Geometry check sheet. Reference: the model listing, model coordinates, mm. A direction names the side the tool comes from. Give positions to 0.01 mm unless a question says otherwise; leave off trailing zeros. Order: outer loops, then holes, each group sorted by start corner. A loop starts at its lowest first (then second) coordinate and runs counter-clockwise, first axis right, second up. Notation, with made-up numbers: M 65,11 L 80,11 A23 cw 80,40 Z; hole C -18.75,-27.75 d11. An arc over 180 degrees is marked long. Answer as a JSON object with one key per item and string values. Group by question number.
from build123d import *

# Parameters (mm, degrees)
SKETCH1_W            = 72
SKETCH1_H            = 125
BOSS_EXTRUDE1_DEPTH  = 2
SKETCH5_W            = 72
SKETCH5_H            = 2
BOSS_EXTRUDE3_DEPTH  = 35
SKETCH6_W            = 2
SKETCH6_H            = 125
BOSS_EXTRUDE4_DEPTH  = 35
SKETCH7_W            = 5
SKETCH7_H            = 5
BOSS_EXTRUDE5_DEPTH  = 35
FILLET2_R            = 1.5
SKETCH8_R            = 2.375
CUT_EXTRUDE2_DEPTH   = 92.049437121
FILLET2_OF_MIRROR4_R = 1.5
FILLET3_R            = 2
SKETCH12_W           = 68
SKETCH12_H           = 2
BOSS_EXTRUDE6_DEPTH  = 35
SKETCH13_W           = 5
SKETCH13_H           = 5
BOSS_EXTRUDE9_DEPTH  = 35
SKETCH14_R           = 2.375
CUT_EXTRUDE6_DEPTH   = 92.049437121
FILLET4_R            = 1.5
FILLET4_OF_MIRROR8_R = 1.5


with BuildPart() as part:
    # Sketch1 → Boss-Extrude1 (new body)
    with BuildSketch(Plane.XY):
        with Locations((0, -12.5)):
            Rectangle(SKETCH1_W, SKETCH1_H)
    extrude(amount=BOSS_EXTRUDE1_DEPTH)

    # Sketch5 → Boss-Extrude3 (add)
    with BuildSketch(Plane.XY.offset(2)):
        with Locations((0, 49)):
            Rectangle(SKETCH5_W, SKETCH5_H)
    extrude(amount=BOSS_EXTRUDE3_DEPTH)

    # Sketch6 → Boss-Extrude4 (add)
    with BuildSketch(Plane.XY.offset(2)):
        with Locations((-35, -12.5)):
            Rectangle(SKETCH6_W, SKETCH6_H)
    boss_extrude4 = extrude(amount=BOSS_EXTRUDE4_DEPTH)

    # Mirror2: Boss-Extrude4 across plane
    add(boss_extrude4.mirror(Plane(origin=(0, 0, 0), x_dir=(0, 0, 1), z_dir=(1, 0, 0))))

    # Sketch7 → Boss-Extrude5 (add)
    with BuildSketch(Plane.XY.offset(2)):
        with Locations((-31.5, 45.5)):
            Rectangle(SKETCH7_W, SKETCH7_H)
    boss_extrude5 = extrude(amount=BOSS_EXTRUDE5_DEPTH)

    # Fillet2
    fillet2_edges = [part.edges().sort_by_distance(p)[0] for p in [
        (-29, 43, 19.5),
    ]]
    fillet(fillet2_edges, radius=FILLET2_R)

    # Sketch8 → Cut-Extrude2 (cut, through all)
    with BuildSketch(Plane.XY.offset(37)):
        with Locations((-32.2, 46.2)):
            Circle(SKETCH8_R)
    cut_extrude2 = extrude(amount=-CUT_EXTRUDE2_DEPTH, mode=Mode.SUBTRACT)

    # Mirror4: Boss-Extrude5, Cut-Extrude2 across plane
    add(boss_extrude5.mirror(Plane(origin=(0, 0, 0), x_dir=(0, 0, 1), z_dir=(1, 0, 0))))
    add(cut_extrude2.mirror(Plane(origin=(0, 0, 0), x_dir=(0, 0, 1), z_dir=(1, 0, 0))), mode=Mode.SUBTRACT)

    # Fillet2 of Mirror4
    fillet2_of_mirror4_edges = [part.edges().sort_by_distance(p)[0] for p in [
        (29, 43, 19.5),
    ]]
    fillet(fillet2_of_mirror4_edges, radius=FILLET2_OF_MIRROR4_R)

    # Fillet3
    fillet3_edges = [part.edges().sort_by_distance(p)[0] for p in [
        (-36, 50, 18.5),
        (36, 50, 18.5),
        (-36, -75, 18.5),
        (36, -75, 18.5),
    ]]
    fillet(fillet3_edges, radius=FILLET3_R - 0.0001)  # a hair under: the kernel refuses the full size

    # Sketch12 → Boss-Extrude6 (add)
    with BuildSketch(Plane.XY.offset(2)):
        with Locations((0, -74)):
            Rectangle(SKETCH12_W, SKETCH12_H)
    extrude(amount=BOSS_EXTRUDE6_DEPTH)

    # Sketch13 → Boss-Extrude9 (add)
    with BuildSketch(Plane.XY.offset(37)):
        with Locations((-31.5, -70.5)):
            Rectangle(SKETCH13_W, SKETCH13_H)
    boss_extrude9 = extrude(amount=-BOSS_EXTRUDE9_DEPTH)

    # Sketch14 → Cut-Extrude6 (cut, through all)
    with BuildSketch(Plane.XY.offset(37)):
        with Locations((-32.2, -71.2)):
            Circle(SKETCH14_R)
    cut_extrude6 = extrude(amount=-CUT_EXTRUDE6_DEPTH, mode=Mode.SUBTRACT)

    # Fillet4
    fillet4_edges = [part.edges().sort_by_distance(p)[0] for p in [
        (-29, -68, 19.5),
    ]]
    fillet(fillet4_edges, radius=FILLET4_R)

    # Mirror8: Boss-Extrude9, Cut-Extrude6 across plane
    add(boss_extrude9.mirror(Plane(origin=(0, 0, 0), x_dir=(0, 0, 1), z_dir=(1, 0, 0))))
    add(cut_extrude6.mirror(Plane(origin=(0, 0, 0), x_dir=(0, 0, 1), z_dir=(1, 0, 0))), mode=Mode.SUBTRACT)

    # Fillet4 of Mirror8
    fillet4_of_mirror8_edges = [part.edges().sort_by_distance(p)[0] for p in [
        (29, -68, 19.5),
    ]]
    fillet(fillet4_of_mirror8_edges, radius=FILLET4_OF_MIRROR8_R)


solid = part.part
1. Cross-section at C-C (z = 23). Record the cut outline in (x, y) (3 decimals), and give its area (3 significant figures).
2. Release check for a two-part mould opening along X. For faces 1 (the flat face through (-36, -13, 18)), 2 (the flat face through (36, -13, 18)), 3 (the cylindrical face through (30.92, -69.2, 18.76)), 4 (the flat face through (0, 50, 18)) record: released by +X, released by -X, zero draft, split by the parting line, or undercut.
3. Cross-section at B-B (x = 32.2). Record the cut outline in (y, z) (3 decimals).
4. Cross-section at D-D (x = 20). Record the cut outline in (y, z).
5. Access from +Z, -Z, +X, -X, +Y, -Y to the whole of each face (thin tool, end or side, straight path). Record for faces 5 (the cylindrical face through (-30.92, -69.2, 18.76)), 6 (the flat face through (34, -13, 19)).
6. Thickness scan on line 1 along Y through (x, z) = (-32.2, 23) (3 decimals); line 2 along X through (y, z) = (-59, 19); line 3 along Y through (x, z) = (-15.5, 11). Record the ranges inside material, lowest first. Write a range as [from, to].
7. Depth check by flat-ended pin: pin 1 (20.5 mm diameter, centred on x = -1.5, y = -8, fed in from +Z). Enter the tip coordinate at first touch or a pass-through.
8. Cross-section at A-A (y = -71.2). Record the cut outline in (x, z) (3 decimals).
Report:
{
 "1": {"outline": "M -36,-73 A2 ccw -34,-75 L 34,-75 A2 ccw 36,-73 L 36,48 A2 ccw 34,50 L -34,50 A2 ccw -36,48 Z; hole C -32.2,-71.2 d4.75; hole C -32.2,46.2 d4.75; hole M -34,-68 L -30.5,-68 A1.5 cw -29,-69.5 L -29,-73 L 29,-73 L 29,-69.5 A1.5 cw 30.5,-68 L 34,-68 L 34,43 L 30.5,43 A1.5 cw 29,44.5 L 29,48 L -29,48 L -29,44.5 A1.5 cw -30.5,43 L -34,43 Z; hole C 32.2,-71.2 d4.75; hole C 32.2,46.2 d4.75", "area": "796 mm2"},
 "2": {"face 1": "released by -X", "face 2": "released by +X", "face 3": "undercut", "face 4": "zero draft"},
 "3": {"outline": "M -75,0 L -73.575,0 L -73.575,37 L -75,37 Z; M -68.825,0 L 43.825,0 L 43.825,37 L 43,37 L 43,2 L -68,2 L -68,37 L -68.825,37 Z; M 48.575,0 L 50,0 L 50,37 L 48.575,37 Z"},
 "4": {"outline": "M -75,0 L 50,0 L 50,37 L 48,37 L 48,2 L -73,2 L -73,37 L -75,37 Z"},
 "5": {"face 5": "+Z, -Z", "face 6": "+Z"},
 "6": {"line 1": "y = [-75, -73.575], [-68.825, -68], [43, 43.825], [48.575, 50]", "line 2": "x = [-36, -34], [34, 36]", "line 3": "y = [-75, -73], [48, 50]"},
 "7": {"pin 1": "stops at z = 2"},
 "8": {"outline": "M -36,0 L -34.575,0 L -34.575,37 L -36,37 Z; M -29.825,0 L 29.825,0 L 29.825,37 L 29,37 L 29,2 L -29,2 L -29,37 L -29.825,37 Z; M 34.575,0 L 36,0 L 36,37 L 34.575,37 Z"}
}
